from build123d import *

# Parameters (mm, degrees)
F1_DEPTH    = 2
F2_DEPTH    = 15
F3_T1_DEPTH = 65.3920789545
F3_T3_DEPTH = 65.4809656857


# Not quite as in the source:
# - a fillet or chamfer that OpenCascade refuses, or shapes differently, is made with other operations: its cross-section is extruded or revolved along the edge and cut away or added


with BuildPart() as f1:
    # F0 (on Top) → F1 (new body)
    with BuildSketch(Plane.XY):
        Polygon((6.2144221197, 1.7468538459), (-7.3403550955, 9.487123932), (-4.5410526356, -5.9592496019), align=None)
        Polygon((9.1590517926, 0.0653633566), (6.2144221197, 1.7468538459), (-4.5410526356, -5.9592496019), (-3.9522281139, -9.2083459887), align=None)
    extrude(amount=F1_DEPTH)

    # F0 (on Top) → F2 (join)
    with BuildSketch(Plane.XY):
        Polygon((9.1590517926, 0.0653633566), (6.2144221197, 1.7468538459), (-4.5410526356, -5.9592496019), (-3.9522281139, -9.2083459887), align=None)
    extrude(amount=F2_DEPTH)

    # F3: chamfer of 12 x 6.9282032303 on 2 edges, made by hand

    # F3_s2 → F3_t1 (cut)
    with BuildSketch(Plane(origin=(-4.6347910576, 25.5744832693, 0), x_dir=(0, 0, 1), z_dir=(0.1783224727, -0.9839721011, 0))):
        Polygon((3, 5.5309372275), (15, -1.3972660027), (15, 5.5309372275), align=None)
    extrude(amount=F3_T1_DEPTH, mode=Mode.SUBTRACT)

    # F3_s4 → F3_t3 (cut)
    with BuildSketch(Plane(origin=(33.8378902633, -19.3226642995, 0), x_dir=(0, 0, 1), z_dir=(-0.8683898362, 0.4958821356, 0))):
        Polygon((15, -2.3296321932), (3, 4.5985710371), (15, 4.5985710371), align=None)
    extrude(amount=F3_T3_DEPTH, mode=Mode.SUBTRACT)


solid = f1.part
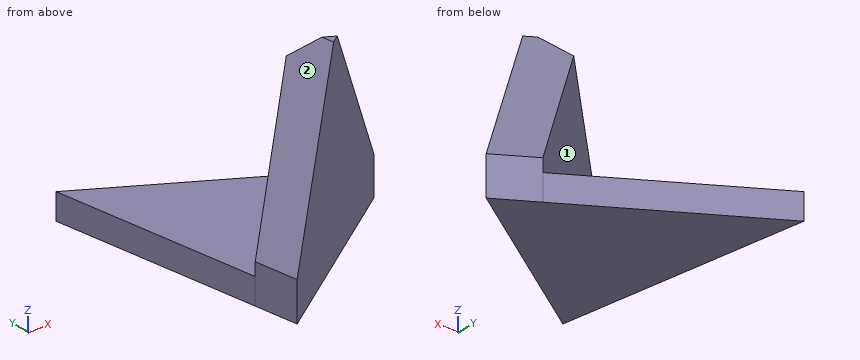
The listing builds one solid part. Answer for the finished solid, in the listing's coordinates (mm). Face numbers are marked on the shaded views. A direction names the side the tool comes from. Give positions to 0.01 mm unless a question says otherwise; leave off trailing zeros. Loops run counter-clockwise (first coordinate to the right, second up) from the corner with the lowest first, then second, coordinate; pieces in that order, holes last. Notation, with made-up numbers: (40.25, -5) - (80.25, -5) arc R18 cw to (80.25, 11) - close; hole circle Ø10 at (-12, 33). An arc over 180 degrees is marked (long way). Use one line per item in the form item = value.
1. Given pin 1 Ø1 at (x, z) = (-5, 3.5) entering from -Y; pin 2 Ø2 at (x, z) = (-0.5, 5.5) entering from +Y; pin 3 Ø6 at (x, y) = (-4, -4) entering from +Z, each flat-ended and moving along its own axis, determine where each tip first touches the part or whether it passes through.
Calculated:
pin_1 = through
pin_2 = -2.35
pin_3 = 9.72
2. Section A-A on z = 1.75 is taken. Give the vertices of the cut face in (x, y), then the cut area to 3 significant figures.
Calculated:
outline = (-7.34, 9.49) - (-3.95, -9.21) - (9.16, 0.07) - close
area = 138 mm^2
3. Section C-C on y = -0.25 is taken. Give the vertices of the cut face in (x, z), then the cut area to 3 significant figures.
Calculated:
outline = (-5.58, 0) - (8.71, 0) - (8.71, 3.86) - (3.43, 8.4) - (3.43, 2) - (-5.58, 2) - close
area = 50.4 mm^2
4. Which of the six approach directions +Z, -Z, +X, -X, +Y, -Y give full straight-line access (tool end or side, diameter ignored) to the marked faces 1 and 2?
Calculated:
face_1 = +Z, -X, +Y
face_2 = +Z, -X, -Y
5. Section B-B on x = -2.25 is taken. Give the vertices of the cut face in (y, z).
Calculated:
outline = (-8, 0) - (6.58, 0) - (6.58, 2) - (-4.32, 2) - (-4.32, 7.41) - (-8, 6.27) - close
6. Section D-D on z = 5.25 is taken. Give the vertices of the cut face in (x, y).
Calculated:
outline = (-3.37, -5.12) - (-2.78, -8.38) - (7.99, -0.76) - (5.05, 0.91) - close
7. Find the intervals of material crossed by line 1 along Z through (x, y) = (3.25, 1.25); line 2 along Y through (x, z) = (4, 5.5); line 3 along Y through (x, z) = (6.5, 5.25), in increasing order. Write a range as [from, to].
Calculated:
line_1 = [0, 2]
line_2 = [-3.58, 0.16]
line_3 = [-1.82, 0.09]
